CAD build for the part. Positions are in the model's coordinates, mm. A direction names the side the tool comes from. Coordinates: 2 decimals unless noted, no trailing zeros.
1) Two-plate mould, pull along Y, no slides. Class faces 1 (the flat face through (0, -15.931, -3)), 2 (the flat face through (-6.557, -23.326, 2.564)), 3 (the flat face through (0, -31.356, -3)): +Y half, -Y half, draft (parallel to the pull), parting line (faces both ways), or undercut.
2) Pin check, flat tips, straight feed: pin 1 Ø4 at (x, z) = (8, 6) entering from +Y; pin 2 Ø6 at (y, z) = (-18, 4) entering from -X; pin 3 Ø3.5 at (x, z) = (-3.5, -4) entering from -Y. Stop position of each tip, or through.
3) Which spindle directions (+Z, -Z, +X, -X, +Y, -Y) get a long thin tool onto all of the face, cutting with end or side? Do faces 4 (the flat face through (-2, -24, -5)), 5 (the flat face through (7, -24, -3)). Say none if no direction does.
4) Wall check: line 1 along Z through (x, y) = (-0.5, -22.5); line 2 along Z through (x, y) = (2.5, -24.5); line 3 along Z through (x, y) = (16, -8). Give the ranges that are in metal, low to high.
```python
from build123d import *

# Parameters (mm, degrees)
BOSS_EXTRUDE1_DEPTH     = 10
SKETCH3_W               = 26.349262508
SKETCH3_H               = 68.843906453
CUT_EXTRUDE1_DEPTH      = 56.145262863
CUT_EXTRUDE1_DEPTH_BACK = 56.145262863
CUT_EXTRUDE2_DEPTH      = 56.002384149
CUT_EXTRUDE2_DEPTH_BACK = 56.002384149
CUT_EXTRUDE4_DEPTH      = 10
CUT_EXTRUDE5_DEPTH      = 46.333254596
CUT_EXTRUDE5_DEPTH_BACK = 46.333254596
BOSS_EXTRUDE2_START     = -5
BOSS_EXTRUDE2_DEPTH     = 13
BOSS_EXTRUDE4_START     = 7
SKETCH11_W              = 3
SKETCH11_H              = 15.425223653
BOSS_EXTRUDE4_DEPTH     = 15


with BuildPart() as part:
    # Sketch2 → Boss-Extrude1 (new body)
    with BuildSketch(Plane.XY):
        with BuildLine():
            ThreePointArc((20.902943543, -1.119068355), (15.061634654, 6.475690428), (8, 0))
            ThreePointArc((8, 0), (0, -8), (-8, 0))
            ThreePointArc((-8, 0), (-15.061634654, 6.475690428), (-20.902943543, -1.119068355))
            add(Edge.make_bspline(
                [(-20.902943543, -1.119068355), (-19.287028044, -26.367706227), (-3.931804619, -48.088836745)],
                knots=[0, 0, 0, 1, 1, 1], degree=2))
            ThreePointArc((-3.931804619, -48.088836745), (0, -50), (3.931804619, -48.088836745))
            add(Edge.make_bspline(
                [(3.931804619, -48.088836745), (19.287028044, -26.367706227), (20.902943543, -1.119068355)],
                knots=[0.990027735, 0.990027735, 0.990027735, 1.990027735, 1.990027735, 1.990027735], degree=2))
        make_face()
    extrude(amount=BOSS_EXTRUDE1_DEPTH)

    # Sketch3 → Cut-Extrude1 (cut, two sides)
    with BuildSketch(Plane(origin=(0, 0, 0), x_dir=(0, 0, -1), z_dir=(1, 0, 0))) as cut_extrude1_sk:
        with Locations((-0.626059786, -22.605093502)):
            Rectangle(SKETCH3_W, SKETCH3_H)
        with BuildLine():
            Line((-2.5, 6.5), (0, 6.5))
            add(Edge.make_bspline(
                [(0, 6.5), (-14.408545927, -21.081950651), (0, -50)],
                knots=[0, 0, 0, 1, 1, 1], degree=2))
            Line((0, -50), (-2.5, -50))
            add(Edge.make_bspline(
                [(-2.5, 6.5), (-10.733514135, -10.976620558), (-12.053907629, -32.649723791), (-2.5, -50)],
                knots=[0, 0, 0, 0, 1, 1, 1, 1], degree=3))
        make_face(mode=Mode.SUBTRACT)
    extrude(amount=CUT_EXTRUDE1_DEPTH, mode=Mode.SUBTRACT)
    extrude(cut_extrude1_sk.sketch, amount=-CUT_EXTRUDE1_DEPTH_BACK, mode=Mode.SUBTRACT)

    # Sketch6 → Cut-Extrude2 (cut, two sides)
    with BuildSketch(Plane.XY) as cut_extrude2_sk:
        with BuildLine():
            Line((-9.557408926, -39.200378686), (-14.826233878, -49.923840658))
            Line((-14.826233878, -49.923840658), (21.939629108, -53.600426957))
            Line((21.939629108, -53.600426957), (9.557408926, -39.200378686))
            add(Edge.make_bspline(
                [(-9.557408926, -39.200378686), (-5.942899698, -46.006320571), (5.857464148, -45.921239034), (9.557408926, -39.200378686)],
                knots=[0, 0, 0, 0, 1, 1, 1, 1], degree=3))
        make_face()
    extrude(amount=CUT_EXTRUDE2_DEPTH, mode=Mode.SUBTRACT)
    extrude(cut_extrude2_sk.sketch, amount=-CUT_EXTRUDE2_DEPTH_BACK, mode=Mode.SUBTRACT)

    # Sketch8 → Cut-Extrude4 (cut)
    with BuildSketch(Plane.XY):
        with BuildLine():
            Line((-13.816005164, -30.617040202), (-11.76409894, -45.724796066))
            Line((-11.76409894, -45.724796066), (9.724502839, -47.837234885))
            Line((9.724502839, -47.837234885), (13.816005164, -30.617040202))
            add(Edge.make_bspline(
                [(-13.816005164, -30.617040202), (-9.778124174, -41.160624176), (10.772333276, -42.703617762), (13.816005164, -30.617040202)],
                knots=[0, 0, 0, 0, 1, 1, 1, 1], degree=3))
        make_face()
    extrude(amount=CUT_EXTRUDE4_DEPTH, mode=Mode.SUBTRACT)

    # Sketch9 → Cut-Extrude5 (cut, two sides)
    with BuildSketch(Plane.XY) as cut_extrude5_sk:
        with BuildLine():
            Line((-28.08585552, 3.22203692), (-20.178308463, -8.029241074))
            ThreePointArc((-20.178308463, -8.029241074), (-15.362673917, -0.358132046), (-7.0095805, -3.859857359))
            Line((-7.0095805, -3.859857359), (-4.822672945, -1.298112458))
            Line((-4.822672945, -1.298112458), (-10.044224813, 8.365655178))
            Line((-10.044224813, 8.365655178), (-28.08585552, 3.22203692))
        make_face()
    extrude(amount=CUT_EXTRUDE5_DEPTH, mode=Mode.SUBTRACT)
    extrude(cut_extrude5_sk.sketch, amount=-CUT_EXTRUDE5_DEPTH_BACK, mode=Mode.SUBTRACT)

    # Sketch10 → Boss-Extrude2 (add)
    with BuildSketch(Plane.XY.offset(BOSS_EXTRUDE2_START)):
        Polygon((-7.615886076, -15.930661374), (-5.468083043, -30.930661374), (-8.437794283, -31.355885027), (-10.585597315, -16.355885027), align=None)
    extrude(amount=BOSS_EXTRUDE2_DEPTH)

    # Sketch11 → Boss-Extrude4 (add)
    with BuildSketch(Plane(origin=(0, 0, 0), x_dir=(0, 0, -1), z_dir=(1, 0, 0)).offset(BOSS_EXTRUDE4_START)):
        with Locations((3.5, -23.643273201)):
            Rectangle(SKETCH11_W, SKETCH11_H)
    extrude(amount=-BOSS_EXTRUDE4_DEPTH)


solid = part.part
```
Data:
1. face 1: +Y half
1. face 2: undercut
1. face 3: -Y half
2. pin 1: stops at y = 2.82
2. pin 2: stops at x = -10.59
2. pin 3: stops at y = -31.36
3. face 4: -Z, +X, -X, +Y, -Y
3. face 5: -Z, +X, +Y, -Y
4. line 1: z = -5 to -2, 7.19 to 9.18
4. line 2: z = -5 to -2, 7.12 to 9.16
4. line 3: z = 5.56 to 7.49
